Part model, mm, in its own coordinate system. A direction names the side the tool comes from. Round coordinates to 2 decimals unless told otherwise and drop trailing zeros. Loops run counter-clockwise (first coordinate to the right, second up) from the corner with the lowest first, then second, coordinate; pieces in that order, holes last. Notation, with made-up numbers: (17, -30.5) -> (51, -30.5) arc R9 cw to (51, -19.5) -> close; hole circle Ø7 at (-39, 28). An arc over 180 degrees is marked (long way). Answer as CSV lines item,"result".
from build123d import *

# Parameters (mm, degrees)
SKETCH_W     = 20
SKETCH_H     = 20
PAD_DEPTH    = 4
SKETCH001_W  = 10
SKETCH001_H  = 20
PAD001_DEPTH = 13
SKETCH002_R  = 3.4
PAD002_DEPTH = 16
SKETCH003_R  = 3.5
POCKET_DEPTH = 16.2


with BuildPart() as part:
    # Sketch → Pad (new body)
    with BuildSketch(Plane.XY):
        Rectangle(SKETCH_W, SKETCH_H)
    extrude(amount=PAD_DEPTH)

    # Sketch001 → Pad001 (new body)
    with BuildSketch(Plane.XY.offset(4)):
        with Locations((5, 0)):
            Rectangle(SKETCH001_W, SKETCH001_H)
    extrude(amount=PAD001_DEPTH)

    # Sketch002 → Pad002 (new body)
    with BuildSketch(Plane.XY.offset(4)):
        with Locations((-4.5, 5)):
            Circle(SKETCH002_R)
        Polygon((-8.5, -5), (-2.5, -1.535898), (-2.5, -8.464102), align=None)
    extrude(amount=PAD002_DEPTH)

    # Sketch003 → Pocket (cut)
    with BuildSketch(Plane.XY.offset(17)):
        with Locations((4.5, 5)):
            Circle(SKETCH003_R)
        Polygon((2.433333, -1.420428), (2.433333, -8.579572), (8.633333, -5), align=None)
    extrude(amount=-POCKET_DEPTH, mode=Mode.SUBTRACT)


solid = part.part
Q1. Drill centre lines: line 1 along X through (y, z) = (-7.5, 12.25); line 2 along X through (y, z) = (5.5, 5.5); line 3 along Y through (x, z) = (4.5, 11.25). Where is each one in solid material? Low to high.
Geometry results:
line 1,"-4.17 to -2.5, 0 to 2.43, 4.3 to 10"
line 2,"-7.86 to -1.14, 0 to 1.04, 7.96 to 10"
line 3,"-10 to -7.39, -2.61 to 1.5, 8.5 to 10"
Q2. Saw through at D-D, the plane x = -4.5. Write the cut outline in (y, z), then the cut area to 3 significant figures.
Geometry results:
outline,"(-10, 0) -> (10, 0) -> (10, 4) -> (8.4, 4) -> (8.4, 20) -> (1.6, 20) -> (1.6, 4) -> (-2.69, 4) -> (-2.69, 20) -> (-7.31, 20) -> (-7.31, 4) -> (-10, 4) -> close"
area,"263 mm2"
Q3. Two-plate mould, pull along X, no slides. Class faces 1 (the face through (-5, 0, 4)), 2 (the face through (7.733, 3.659, 9.013)), 3 (the face through (-5.458, -6.756, 11.888)), 4 (the face through (4, -10, 6)): pulls with the +X half, pulls with the -X half, needs draft (parallel to the pull), parting line crosses it, or undercut.
Geometry results:
face 1,"undercut"
face 2,"undercut"
face 3,"pulls with the -X half"
face 4,"needs draft"
Q4. Saw through at C-C, the plane z = 17.75. Write the cut outline in (x, y), then the cut area to 3 significant figures.
Geometry results:
outline,"(-8.5, -5) -> (-2.5, -8.46) -> (-2.5, -1.54) -> close; circle Ø6.8 at (-4.5, 5)"
area,"57.1 mm2"
Q5. Which spindle directions (+Z, -Z, +X, -X, +Y, -Y) get a long thin tool onto all of the face, cutting with end or side? Do faces 5 (the face through (-2.5, -5, 12)), 6 (the face through (5, 0, 17)), 7 (the face through (0, 0, 10)), 8 (the face through (5.49, -6.815, 9.013)). Say none if no direction does.
Geometry results:
face 5,"+Z, -Y"
face 6,"+Z, +X, +Y, -Y"
face 7,"+Z, +Y, -Y"
face 8,"+Z"
Q6. Saw through at A-A, the plane z = 15.75. Write the cut outline in (x, y).
Geometry results:
outline,"(-8.5, -5) -> (-2.5, -8.46) -> (-2.5, -1.54) -> close; circle Ø6.8 at (-4.5, 5); (0, -10) -> (10, -10) -> (10, 10) -> (0, 10) -> close; hole circle Ø7 at (4.5, 5); hole (2.43, -8.58) -> (8.63, -5) -> (2.43, -1.42) -> close"
Q7. Saw through at B-B, the plane y = -0.25. Write the cut outline in (x, z).
Geometry results:
outline,"(-10, 0) -> (10, 0) -> (10, 17) -> (0, 17) -> (0, 4) -> (-10, 4) -> close"
Q8. Drop flat-ended pins along their axis: P1, Ø3, axis at x = 6.5, y = -5, coming from the +Z side; P2, Ø4, axis at y = -2.5, z = 13.5, coming from the -X side; P3, Ø6.5, axis at y = -2, z = 13, coming from the -X side. Give the stop position or say it passes through.
Geometry results:
P1,"z = 17"
P2,"x = -7.63"
P3,"x = -8.5"
